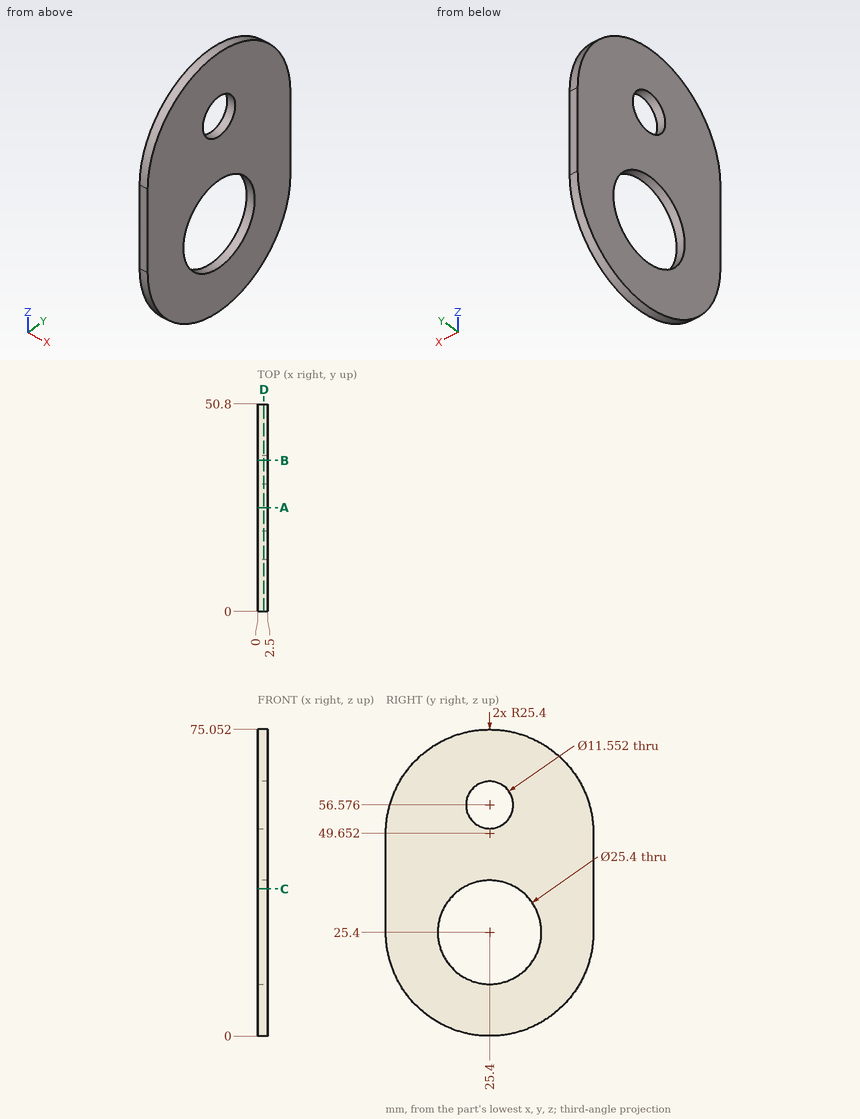
The figure shows three views and two pictorial views of one solid part (mm, origin at its lowest corner). Answer the questions. Round coordinates to 2 decimals unless told otherwise and drop trailing zeros. Loops run counter-clockwise (first coordinate to the right, second up) from the corner with the lowest first, then second, coordinate; pieces in that order, holes last. Notation, with made-up numbers: (53.5, 32) - (98.5, 32) arc R15 ccw to (98.5, 57) - close; hole circle Ø4 at (65.25, 29.25). An arc over 180 degrees is marked (long way). Use one line per item in the form item = value. Start each with the question number.
(1) Find section A-A on y = 25.4. Determine the outline of the cut face in (x, z).
(2) Flat-ended cylindrical pins translate along their axes: P1, Ø1, axis at x = 1, z = 62.5, coming from the -Y side; P2, Ø1.5, axis at x = 1, z = 19, coming from the -Y side. Find the tip coordinate at first contact, or state that the pin passes through.
(3) Find section C-C on z = 36. Determine the outline of the cut face in (x, y) (3 decimals), and give its area (3 significant figures).
(4) Find section B-B on y = 37. Determine the outline of the cut face in (x, z), and give its area (3 significant figures).
(5) Find section D-D on x = 1.5. Determine the outline of the cut face in (y, z).
(6) Consider line 1 (Z direction, x = 0.65, y = 25.4); line 2 (Z direction, x = 1.3, y = 25); line 3 (Y direction, x = 0.85, z = 25.4). Determine where each line is inside the solid, lowest interval first.
Answer list:
q1.outline = (0, 0) - (2.5, 0) - (2.5, 12.7) - (0, 12.7) - close; (0, 38.1) - (2.5, 38.1) - (2.5, 50.8) - (0, 50.8) - close; (0, 62.35) - (2.5, 62.35) - (2.5, 75.05) - (0, 75.05) - close
q2.P1 = 3.2
q2.P2 = 0.64
q3.outline = (0, 0) - (2.5, 0) - (2.5, 18.405) - (0, 18.405) - close; (0, 32.395) - (2.5, 32.395) - (2.5, 50.8) - (0, 50.8) - close
q3.area = 92.0 mm^2
q4.outline = (0, 2.8) - (2.5, 2.8) - (2.5, 20.23) - (0, 20.23) - close; (0, 30.57) - (2.5, 30.57) - (2.5, 72.25) - (0, 72.25) - close
q4.area = 148 mm^2
q5.outline = (0, 25.4) arc R25.4 ccw to (50.8, 25.4) - (50.8, 49.65) arc R25.4 ccw to (0, 49.65) - close; hole circle Ø25.4 at (25.4, 25.4); hole circle Ø11.55 at (25.4, 56.58)
q6.line_1 = 0 to 12.7, 38.1 to 50.8, 62.35 to 75.05
q6.line_2 = 0 to 12.71, 38.09 to 50.81, 62.34 to 75.05
q6.line_3 = 0 to 12.7, 38.1 to 50.8
